Can you work these out from the model? Positions are in its coordinate system, mm. Face numbers are marked on the shaded views. Give positions to 0.01 mm unless a question says otherwise; leave off trailing zeros. Order: outer loops, then holes, each group sorted by start corner. A loop starts at its lowest first (then second) coordinate and runs counter-clockwise, first axis right, second up. Notation, with made-up numbers: (9, 78) -> (66, 78) arc R17 cw to (66, 83) -> close; hole circle Ø11 at (51.25, 16). An arc over 180 degrees is marked (long way). Answer as a JSON object with one key per item and string values.
```python
from build123d import *

# Parameters (mm, degrees)
SKETCH1_W           = 25
SKETCH1_H           = 25
SKETCH1_W_2         = 23
SKETCH1_H_2         = 23
BOSS_EXTRUDE1_DEPTH = 200


with BuildPart() as part:
    # Sketch1 → Boss-Extrude1 (new body)
    with BuildSketch(Plane(origin=(0, 0, 0), x_dir=(1, 0, 0), z_dir=(0, 1, 0))):
        Rectangle(SKETCH1_W, SKETCH1_H)
        Rectangle(SKETCH1_W_2, SKETCH1_H_2, mode=Mode.SUBTRACT)
    extrude(amount=BOSS_EXTRUDE1_DEPTH)

    # Sketch2 → Revolve1 (revolve)
    with BuildSketch(Plane(origin=(0, -10, 0), x_dir=(-1, 0, 0), z_dir=(0, -1, 0))):
        with BuildLine():
            Line((0, 19), (0, 20))
            ThreePointArc((0, 20), (-20, 0), (0, -20))
            Line((0, -20), (0, -19))
            ThreePointArc((0, -19), (-19, 0), (0, 19))
        make_face()
    revolve(axis=Axis((0, -10, -20), (0, 0, 1)))


solid = part.part
```
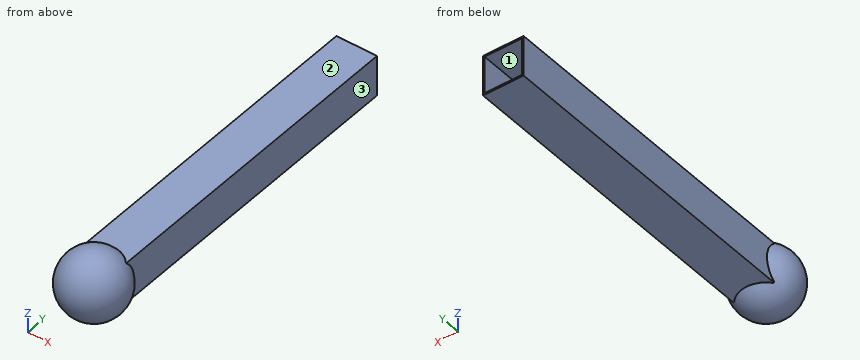
1. If we section it at C-C on x = 3: Please give me the cut outline in (y, z), then the cut area to 3 significant figures.
Worked answers:
{"outline": "(5.32, -12.5) -> (200, -12.5) -> (200, -11.5) -> (6.09, -11.5) arc R19.77 ccw to (6.09, 11.5) -> (200, 11.5) -> (200, 12.5) -> (5.32, 12.5) arc R19.77 ccw (long way) to start; hole (0, -12.5) -> (0, -11.5) -> (4.82, -11.5) arc R18.76 ccw to (4.82, 11.5) -> (0, 11.5) -> (0, 12.5) -> (3.99, 12.5) arc R18.76 ccw (long way) to (3.99, -12.5) -> close", "area": "520 mm²"}
2. If we section it at A-A on y = 163.5: Please give me the cut outline in (x, z).
Worked answers:
{"outline": "(-12.5, -12.5) -> (12.5, -12.5) -> (12.5, 12.5) -> (-12.5, 12.5) -> close; hole (-11.5, -11.5) -> (11.5, -11.5) -> (11.5, 11.5) -> (-11.5, 11.5) -> close"}
3. Will these pins go through, and if not, where does the flat tip stop? pin 1 Ø4 at (x, y) = (-14, 129.5) entering from -Z; pin 2 Ø3.5 at (y, z) = (1.5, -2.5) entering from +X; pin 3 Ø5 at (x, z) = (3.5, -4.5) entering from -Y.
Worked answers:
{"pin 1": "z = -12.5", "pin 2": "x = 17.31", "pin 3": "y = -29.74"}
4. If we section it at B-B on z = 5.5: Please give me the cut outline in (x, y).
Worked answers:
{"outline": "(-12.5, 4.61) arc R19.23 ccw (long way) to (12.5, 4.61) -> (12.5, 200) -> (11.5, 200) -> (11.5, 5.41) arc R19.23 ccw to (-11.5, 5.41) -> (-11.5, 200) -> (-12.5, 200) -> close; hole (-12.5, 0) -> (-12.5, 3.21) arc R18.19 ccw (long way) to (12.5, 3.21) -> (12.5, 0) -> (11.5, 0) -> (11.5, 4.09) arc R18.19 ccw to (-11.5, 4.09) -> (-11.5, 0) -> close"}
5. If we section it at D-D on z = 15.5: Please give me the cut outline in (x, y), then the cut area to 3 significant figures.
Worked answers:
{"outline": "circle Ø25.28 at (0, -10); hole circle Ø21.98 at (0, -10)", "area": "123 mm²"}
6. If we mould it in two halves opening along Z, with no side actions, what happens to the marked faces 1, 2 and 3? For each: +Z half, -Z half, draft (parallel to the pull), parting line (faces both ways), or undercut.
Worked answers:
{"face 1": "undercut", "face 2": "+Z half", "face 3": "draft"}
7. Please list where these lines run through material, in increasing order: L1, parallel to Z at x = 4.5, y = 27.5; L2, parallel to X at y = 180, z = -12.
Worked answers:
{"L1": "-12.5 to -11.5, 11.5 to 12.5", "L2": "-12.5 to 12.5"}
